Model file for the job. Use its own axes, mm. A direction names the side the tool comes from. Coordinates: 2 decimals unless noted, no trailing zeros. Order: outer loops, then holes, each group sorted by start corner. A loop starts at its lowest first (then second) coordinate and runs counter-clockwise, first axis right, second up.
from build123d import *

# Parameters (mm, degrees)
SKETCH1_W            = 1044
SKETCH1_H            = 348
BOSS_EXTRUDE1_DEPTH  = 321.9
CHAMFER2_SIZE        = 222
CHAMFER2_SIZE2       = 103.52030011
FILLET1_R            = 100
SCALE1_SCALE         = 0.115
SKETCH175_W          = 20
SKETCH175_H          = 12
BOSS_EXTRUDE12_DEPTH = 25
SKETCH176_W          = 5
SKETCH176_H          = 25
CUT_EXTRUDE1_DEPTH   = 30
SKETCH177_R          = 2
CUT_EXTRUDE2_DEPTH   = 30
CUT_EXTRUDE4_DEPTH   = 25
FILLET3_R            = 4


with BuildPart() as part:
    # Sketch1 → Boss-Extrude1 (new body)
    with BuildSketch(Plane(origin=(0, 0, 0), x_dir=(1, 0, 0), z_dir=(0, 1, 0))):
        Rectangle(SKETCH1_W, SKETCH1_H)
    extrude(amount=BOSS_EXTRUDE1_DEPTH)

    # Chamfer2
    chamfer2_edges = [part.edges().sort_by_distance(p)[0] for p in [
        (522, 321.9, 0),
    ]]
    chamfer2_side = [part.faces().sort_by_distance(p)[0] for p in [
        (0, 321.9, 0),
    ]]
    chamfer(chamfer2_edges, length=CHAMFER2_SIZE, length2=CHAMFER2_SIZE2, reference=chamfer2_side[0])

    # Fillet1
    fillet1_edges = [part.edges().sort_by_distance(p)[0] for p in [
        (-522, 321.9, 0),
        (-522, 0, 0),
        (-522, 160.95, -174),
        (-522, 160.95, 174),
    ]]
    fillet(fillet1_edges, radius=FILLET1_R)


with BuildPart() as part_1:
    # Scale1: scaled about (-4.978902211, 156.372589253, 0)
    add(part.part.scale(SCALE1_SCALE).moved(Location((-4.406328457, 138.389741489, 0))))


with BuildPart() as boss_extrude12_tool:
    # Sketch175 → Boss-Extrude12 (new body)
    with BuildSketch(Plane.XZ.offset(-138.389734505)):
        with Locations((-4.405349795, 0)):
            Rectangle(SKETCH175_W, SKETCH175_H)
    extrude(amount=BOSS_EXTRUDE12_DEPTH)


with BuildPart() as part_2:
    add(part_1.part)


with BuildPart() as part_3:
    # Boss-Extrude12: joined with boss_extrude12_tool
    add(part_2.part.fuse(boss_extrude12_tool.part, tol=0.00001))

    # Sketch176 → Cut-Extrude1 (cut)
    with BuildSketch(Plane(origin=(5.594650205, 0, 0), x_dir=(0, 0, -1), z_dir=(1, 0, 0))):
        with Locations((0, 125.889734505)):
            Rectangle(SKETCH176_W, SKETCH176_H)
    extrude(amount=-CUT_EXTRUDE1_DEPTH, mode=Mode.SUBTRACT)

    # Sketch177 → Cut-Extrude2 (cut)
    with BuildSketch(Plane(origin=(0, 0, -6), x_dir=(-1, 0, 0), z_dir=(0, 0, -1))):
        with Locations((4.405349795, 121.389734505)):
            Circle(SKETCH177_R)
    extrude(amount=-CUT_EXTRUDE2_DEPTH, mode=Mode.SUBTRACT)

    # Sketch179 → Cut-Extrude4 (cut)
    with BuildSketch(Plane.XZ.offset(-113.389734505)):
        Polygon((-14.405349795, 6), (20.594650205, 3.552561582), (20.594650205, -3.552561582), (-14.405349795, -6), (23.594650205, -6), (23.594650205, 6), align=None)
    extrude(amount=-CUT_EXTRUDE4_DEPTH, mode=Mode.SUBTRACT)

    # Fillet3
    # the kernel refuses this fillet: 4 mm, written as the material it takes off along each edge
    with BuildSketch(Plane(origin=(-14.405349795, 138.389734505, -6), x_dir=(0, 0, 1), z_dir=(0, -1, 0))) as fillet3_piece_1:
        with BuildLine():
            CenterArc((4.284048925, -3.922405803), FILLET3_R, 101.30386139, 82.69613861)
            Line((0.293792724, -4.201431698), (0.2139876, -4.207012216))
            Line((0.2139876, -4.207012216), (-0.079805124, -0.005580518))
            Line((-0.079805124, -0.005580518), (0, 0.08))
            ThreePointArc((0, 0.08), (1.75, 0.08), (3.484319021, 0.078448116))
            Line((3.484319021, 0.078448116), (3.5, 0))
        make_face()
    extrude(amount=35.529227915, mode=Mode.SUBTRACT)
    with BuildSketch(Plane(origin=(-14.405349795, 138.389734505, 6), x_dir=(0, 0, -1), z_dir=(0, -1, 0))) as fillet3_piece_2:
        with BuildLine():
            CenterArc((4.284048925, 3.922405803), FILLET3_R, 176, 82.69613861)
            Line((0.293792724, 4.201431698), (0.2139876, 4.207012216))
            Line((0.2139876, 4.207012216), (-0.079805124, 0.005580518))
            Line((-0.079805124, 0.005580518), (0, -0.08))
            ThreePointArc((0, -0.08), (1.75, -0.08), (3.484319021, -0.078448116))
            Line((3.484319021, -0.078448116), (3.5, 0))
        make_face()
    extrude(amount=35.529227915, mode=Mode.SUBTRACT)


solid = part_3.part
Q1. Cut at B-B, the plane z = -0.5. List the corners of the cut face in (x, y).
Established:
outline: (-64.44, 149.89) arc R11.5 ccw to (-52.94, 138.39) - (5.59, 138.39) - (55.62, 138.39) - (55.62, 163.5) - (30.09, 175.41) - (-52.94, 175.41) arc R11.5 ccw to (-64.44, 163.91) - close
Q2. Which spindle directions (+Z, -Z, +X, -X, +Y, -Y) get a long thin tool onto all of the face, cutting with end or side? Do faces 4 (the face through (43.04, 169.37, 0.28)), 5 (the face through (-2.42, 125.71, 5.16)), 6 (the face through (-4, 126, 2.5)). Say none if no direction does.
Established:
face 4: +Z, -Z, +X, +Y
face 5: +Z, +X, -Y
face 6: +X, -X, -Y
Q3. Probe line 1 (Y direction, x = -39, z = -9.5); line 2 (X direction, y = 166.5, z = 3); line 3 (X direction, y = 167, z = 11.5). List the from-to ranges inside material, lowest first.
Established:
line 1: y = 138.39 to 175.41
line 2: x = -64.14 to 49.2
line 3: x = -64.01 to 48.13
Q4. Cut at C-C, the plane x = -38. List the corners of the cut face in (y, z), plus the area to 3 significant figures.
Established:
outline: (138.39, -20.01) - (175.41, -20.01) - (175.41, 20.01) - (138.39, 20.01) - close
area: 1,480 mm2
Q5. Cut at A-A, the plane y = 135. List the corners of the cut face in (x, z), plus the area to 3 significant figures.
Established:
outline: (-14.41, -2.5) arc R4 ccw to (-10.2, -5.71) - (5.59, -4.6) - (5.59, -2.5) - close; (-14.41, 2.5) - (5.59, 2.5) - (5.59, 4.6) - (-10.2, 5.71) arc R4 ccw to start
area: 105 mm2
Q6. Mould opens along Z. For faces 1 (the face through (-4, 126, -2.5)), 2 (the face through (-12.88, 126.06, 4.92)), 3 (the face through (-6.313, 121.99, 3.95)) say: pulls with the +Z half, pulls with the -Z half, needs draft (parallel to the pull), parting line crosses it, or undercut.
Established:
face 1: undercut
face 2: pulls with the +Z half
face 3: needs draft
Q7. Drop flat-ended pins along their axis: P1, Ø1.5, axis at x = 0, z = 0.5, coming from the -Y side; P2, Ø8, axis at y = 138.5, z = -10.5, coming from the -X side; P3, Ø10, axis at x = 35.5, z = -0.5, coming from the +Y side; P4, Ø2.5, axis at x = -4.41, y = 121.39, coming from the +Z side. Give the stop position or say it passes through.
Established:
P1: stops at y = 138.39
P2: stops at x = -61.75
P3: stops at y = 175.22
P4: passes through
Q8. Cut at D-D, the plane z = -13. List the corners of the cut face in (x, y), plus the area to 3 significant figures.
Established:
outline: (-63.52, 145.4) arc R11.5 ccw to (-52.94, 138.39) - (55.62, 138.39) - (55.62, 163.5) - (30.09, 175.41) - (-52.94, 175.41) arc R11.5 ccw to (-63.52, 168.4) - close
area: 4,220 mm2
